Verification items for the finished model (mm, model axes). Face numbers are marked on the shaded views. A direction names the side the tool comes from. Round coordinates to 2 decimals unless told otherwise and drop trailing zeros. Order: outer loops, then holes, each group sorted by start corner. A loop starts at its lowest first (then second) coordinate and runs counter-clockwise, first axis right, second up. Notation, with made-up numbers: (67, -31) -> (79, -31) arc R26 cw to (79, -14) -> close; hole circle Ø4 at (83, 45). An arc over 180 degrees is marked (long way). Return JSON: item names as keys, results as strings. Group by question number.
1) Tool access check on the marked faces 1 and 2. Record the directions out of +Z, -Z, +X, -X, +Y, -Y that give a thin tool (end or side, any length) a straight path to the whole face; none if there is none.
2) Section check D-D on z = 6.5. Enter the section's corners in (x, y), plus the area to 3 significant figures.
3) Depth check by flat-ended pin: pin 1 (1 mm diameter, centred on x = -15.5, z = 8.5, fed in from -Y); pin 2 (4.5 mm diameter, centred on x = -12, y = 148.5, fed in from +Z); pin 3 (1.5 mm diameter, centred on x = -1, y = 158, fed in from +Z). Enter the tip coordinate at first touch or a pass-through.
4) Section check C-C on x = 21. Enter the section's corners in (y, z).
5) Section check A-A on z = 23.5. Enter the section's corners in (x, y), plus the area to 3 significant figures.
6) Section check B-B on y = 158.25. Enter the section's corners in (x, z), plus the area to 3 significant figures.
7) Scan lines: L1, parallel to X at y = 159.15, z = 23.5; L2, parallel to Y at x = 6, z = 13; L3, parallel to Z at x = 12.5, y = 144.5. Record each from-to range of solid material in increasing order.
```python
from build123d import *

# Parameters (mm, degrees)
SKETCH1_W           = 60
SKETCH1_H           = 3
BOSS_EXTRUDE1_DEPTH = 30
SKETCH2_W           = 60
SKETCH2_H           = 3
BOSS_EXTRUDE2_DEPTH = 15
SKETCH3_W           = 20
SKETCH3_H           = 10
CUT_EXTRUDE1_DEPTH  = 46
FILLET1_R           = 3
SKETCH4_R           = 1
CUT_EXTRUDE2_DEPTH  = 10


with BuildPart() as part:
    # Sketch1 → Boss-Extrude1 (new body)
    with BuildSketch(Plane.XY):
        with Locations((0, 158.5)):
            Rectangle(SKETCH1_W, SKETCH1_H)
    extrude(amount=BOSS_EXTRUDE1_DEPTH)

    # Sketch2 → Boss-Extrude2 (add)
    with BuildSketch(Plane.XZ.offset(-157)):
        with Locations((0, 1.5)):
            Rectangle(SKETCH2_W, SKETCH2_H)
    extrude(amount=BOSS_EXTRUDE2_DEPTH)

    # Sketch3 → Cut-Extrude1 (cut, through all)
    with BuildSketch(Plane.XZ.offset(-157)):
        with Locations((0, 25)):
            Rectangle(SKETCH3_W, SKETCH3_H)
    extrude(amount=-CUT_EXTRUDE1_DEPTH, mode=Mode.SUBTRACT)

    # Fillet1
    fillet1_edges = [part.edges().sort_by_distance(p)[0] for p in [
        (30, 158.5, 30),
        (-30, 142, 1.5),
        (30, 142, 1.5),
        (-30, 158.5, 30),
    ]]
    fillet(fillet1_edges, radius=FILLET1_R)

    # Sketch4 → Cut-Extrude2 (cut)
    with BuildSketch(Plane(origin=(0, 160, 0), x_dir=(1, 0, 0), z_dir=(0, 1, 0))):
        with Locations(Location((-21, -23.5, 0), (0, 0, 270))):
            Circle(SKETCH4_R)
        with Locations(Location((-21, -6.5, 0), (0, 0, 270))):
            Circle(SKETCH4_R)
        with Locations(Location((21, -6.5, 0), (0, 0, 270))):
            Circle(SKETCH4_R)
        with Locations(Location((21, -23.5, 0), (0, 0, 270))):
            Circle(SKETCH4_R)
    extrude(amount=-CUT_EXTRUDE2_DEPTH, mode=Mode.SUBTRACT)


solid = part.part
```
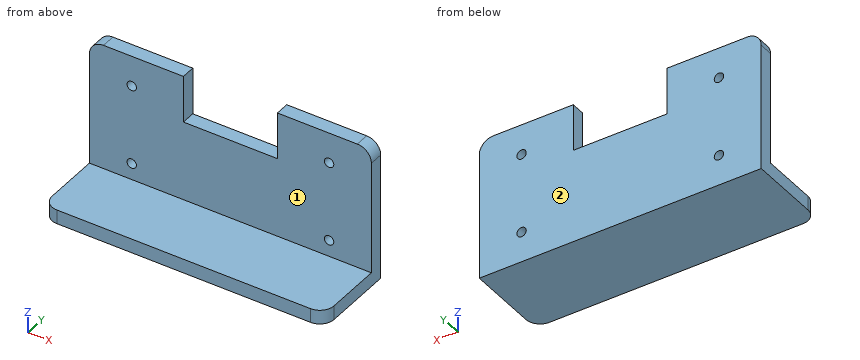
Check result:
{
 "1": {"face 1": "+Z, +X, -X, -Y", "face 2": "+Z, -Z, +X, -X, +Y"},
 "2": {"outline": "(-30, 157) -> (-22, 157) -> (-22, 160) -> (-30, 160) -> close; (-20, 157) -> (20, 157) -> (20, 160) -> (-20, 160) -> close; (22, 157) -> (30, 157) -> (30, 160) -> (22, 160) -> close", "area": "168 mm^2"},
 "3": {"pin 1": "y = 157", "pin 2": "z = 3", "pin 3": "z = 20"},
 "4": {"outline": "(142, 0) -> (160, 0) -> (160, 5.5) -> (157, 5.5) -> (157, 3) -> (142, 3) -> close; (157, 7.5) -> (160, 7.5) -> (160, 22.5) -> (157, 22.5) -> close; (157, 24.5) -> (160, 24.5) -> (160, 30) -> (157, 30) -> close"},
 "5": {"outline": "(-30, 157) -> (-22, 157) -> (-22, 160) -> (-30, 160) -> close; (-20, 157) -> (-10, 157) -> (-10, 160) -> (-20, 160) -> close; (10, 157) -> (20, 157) -> (20, 160) -> (10, 160) -> close; (22, 157) -> (30, 157) -> (30, 160) -> (22, 160) -> close", "area": "108 mm^2"},
 "6": {"outline": "(-30, 0) -> (30, 0) -> (30, 27) arc R3 ccw to (27, 30) -> (10, 30) -> (10, 20) -> (-10, 20) -> (-10, 30) -> (-27, 30) arc R3 ccw to (-30, 27) -> close; hole circle Ø2 at (-21, 6.5); hole circle Ø2 at (-21, 23.5); hole circle Ø2 at (21, 6.5); hole circle Ø2 at (21, 23.5)", "area": "1,580 mm^2"},
 "7": {"L1": "-30 to -22, -20 to -10, 10 to 20, 22 to 30", "L2": "157 to 160", "L3": "0 to 3"}
}
